The figure shows three views and two pictorial views of one solid part (mm, origin at its lowest corner). Answer the questions. A direction names the side the tool comes from. Coordinates: 2 decimals unless noted, no trailing zeros. Write each loop counter-clockwise with the first axis right and the second up, starting at its lowest first coordinate (ties: lowest second). Pieces come first, ordered by that corner, then holes.
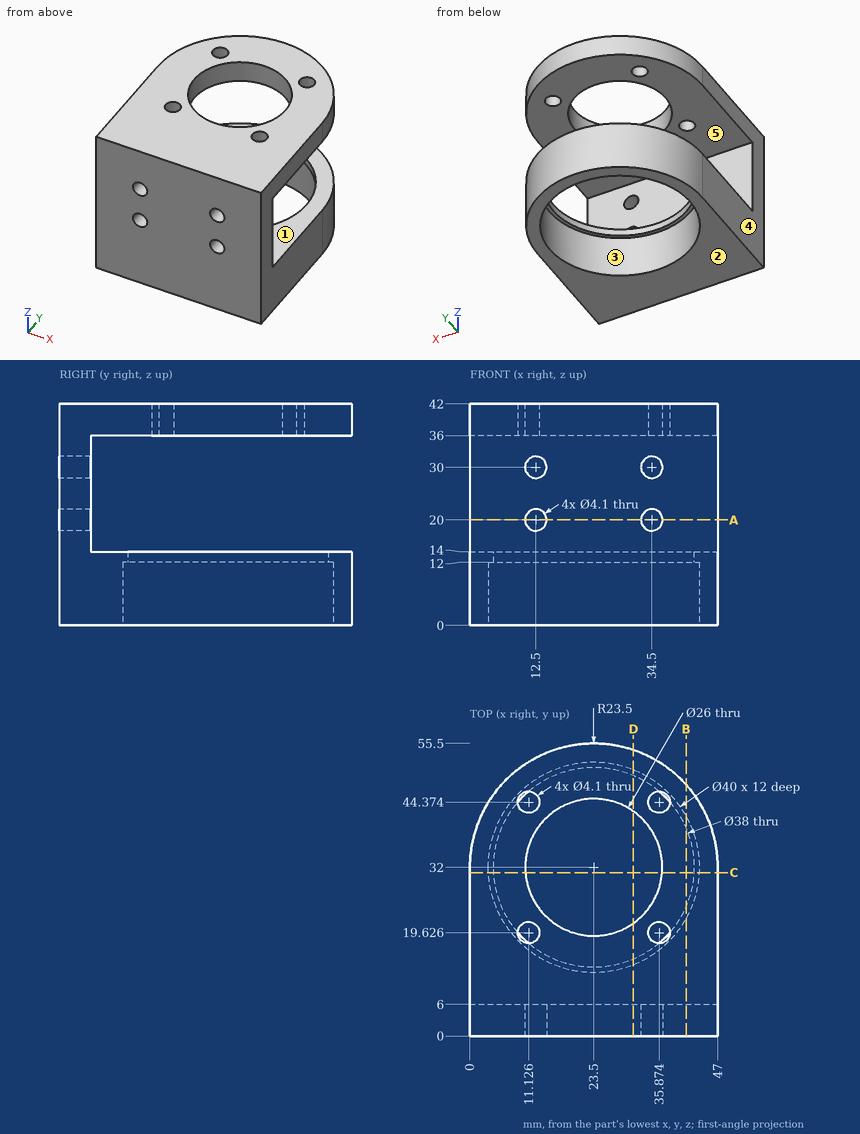
Item 1: For the marked faces 1 and 2, determine the directions among +Z, -Z, +X, -X, +Y, -Y from which every point of the face is accessible in a straight line to the end or side of a thin tool.
Item 2: The part is cut by section A-A (z = 20). Give the vertices of the cut face in (x, y).
Item 3: The part is cut by section D-D (x = 31). Give the vertices of the cut face in (y, z).
Item 4: The part is cut by section C-C (y = 31). Give the vertices of the cut face in (x, z) (1 decimal).
Item 5: The part is cut by section B-B (x = 41). Give the vertices of the cut face in (y, z) (1 decimal), and give its area (3 significant figures).
Item 6: Determine the mould class of the marked faces 3, 4 and 5 for opening direction X: +X half, -X half, draft (parallel to the pull), parting line (faces both ways), or undercut.
Item 7: Find the intervals of material crossed by probe 1 along Z at (x, y) = (12.5, 1.8); probe 2 along X at (y, z) = (3.7, 20); probe 3 along Z at (x, y) = (6, 19.5), in increasing order.
Item 8: Given pin 1 (8 mm diameter, centred on x = 17, z = 16.5, fed in from +Y); pin 2 (3.5 mm diameter, centred on x = 11.13, y = 44.37, fed in from +Z); pin 3 (5.5 mm diameter, centred on x = 11.13, y = 19.63, fed in from +Z); pin 4 (1.5 mm diameter, centred on y = 39.5, z = 5.5, fed in from +X), each flat-ended and moving along its own axis, determine where each tip first touches the part or whether it passes through.
Answer:
1. face 1: +X, -X, +Y
1. face 2: -Z, +X, -X, +Y, -Y
2. outline: (0, 0) - (10.45, 0) - (10.45, 6) - (0, 6) - close; (14.55, 0) - (32.45, 0) - (32.45, 6) - (14.55, 6) - close; (36.55, 0) - (47, 0) - (47, 6) - (36.55, 6) - close
3. outline: (0, 0) - (13.46, 0) - (13.46, 12) - (14.54, 12) - (14.54, 14) - (6, 14) - (6, 36) - (21.38, 36) - (21.38, 42) - (0, 42) - close; (42.62, 36) - (54.27, 36) - (54.27, 42) - (42.62, 42) - close; (49.46, 12) - (50.54, 12) - (50.54, 0) - (54.27, 0) - (54.27, 14) - (49.46, 14) - close
4. outline: (0, 0) - (3.5, 0) - (3.5, 12) - (4.5, 12) - (4.5, 14) - (0, 14) - close; (0, 36) - (10.5, 36) - (10.5, 42) - (0, 42) - close; (36.5, 36) - (47, 36) - (47, 42) - (36.5, 42) - close; (42.5, 12) - (43.5, 12) - (43.5, 0) - (47, 0) - (47, 14) - (42.5, 14) - close
5. outline: (0, 0) - (22.3, 0) - (22.3, 12) - (24.6, 12) - (24.6, 14) - (6, 14) - (6, 36) - (47.7, 36) - (47.7, 42) - (0, 42) - close; (39.4, 12) - (41.7, 12) - (41.7, 0) - (47.7, 0) - (47.7, 14) - (39.4, 14) - close
5. area: 824 mm2
6. face 3: undercut
6. face 4: -X half
6. face 5: draft
7. probe 1: z = 0 to 17.95, 22.05 to 27.95, 32.05 to 42
7. probe 2: x = 0 to 10.45, 14.55 to 32.45, 36.55 to 47
7. probe 3: z = 0 to 14, 36 to 42
8. pin 1: stops at y = 55.26
8. pin 2: stops at z = 14
8. pin 3: stops at z = 42
8. pin 4: stops at x = 46.01
